Check sheet for the modelled part. Datum: model origin and axes. Units: mm. Face numbers are marked on the shaded views. A direction names the side the tool comes from. Coordinates: 2 decimals unless noted, no trailing zeros. Write each loop counter-clockwise with the first axis right and the second up, starting at its lowest first coordinate (ties: lowest second). Pieces come first, ordered by that corner, then holes. Notation, with made-up numbers: (74.5, 49) -> (109.5, 49) arc R13 ccw to (109.5, 56) -> close; hole circle Ø1 at (87.5, -4). An arc over 180 degrees is marked (long way). Put each result on its own line as item: value.
```python
from build123d import *

# Parameters (mm, degrees)
SKETCH033_W     = 136
SKETCH033_H     = 30
PAD012_DEPTH    = 10
SKETCH032_W     = 15
SKETCH032_H     = 30
PAD011_DEPTH    = 22
SKETCH030_W     = 30
SKETCH030_H     = 17
POCKET020_DEPTH = 10
SKETCH031_R     = 3
POCKET021_DEPTH = 10.001
SKETCH034_W     = 32.5
SKETCH034_H     = 30
POCKET022_DEPTH = 5
SKETCH040_R     = 5
POCKET028_DEPTH = 3
CHAMFER_SIZE2   = 25
CHAMFER_SIZE    = 10
CHAMFER010_SIZE = 1
SKETCH080_W     = 32.5
SKETCH080_H     = 9.75
PAD031_DEPTH    = 1
SKETCH084_R     = 3
POCKET051_DEPTH = 5


with BuildPart() as part:
    # Sketch033 → Pad012 (new body)
    with BuildSketch(Plane.XY):
        Rectangle(SKETCH033_W, SKETCH033_H)
    extrude(amount=PAD012_DEPTH)

    # Sketch032 (on Face5 of Pad012) → Pad011 (join)
    with BuildSketch(Plane(origin=(0, 0, 0), x_dir=(1, 0, 0), z_dir=(0, 0, -1))):
        with Locations((-60.5, 0)):
            Rectangle(SKETCH032_W, SKETCH032_H)
    extrude(amount=PAD011_DEPTH)

    # Sketch030 (on Face9 of Pad011) → Pocket020 (cut)
    with BuildSketch(Plane.YZ.offset(-53)):
        with Locations((0, -8.5)):
            Rectangle(SKETCH030_W, SKETCH030_H)
    extrude(amount=-POCKET020_DEPTH, mode=Mode.SUBTRACT)

    # Sketch031 (on Face5 of Pocket020) → Pocket021 (cut, through all)
    with BuildSketch(Plane(origin=(0, 0, 0), x_dir=(1, 0, 0), z_dir=(0, 0, -1))):
        with Locations((53, 0)):
            Circle(SKETCH031_R)
    extrude(amount=-POCKET021_DEPTH, mode=Mode.SUBTRACT)

    # Sketch034 → Pocket022 (cut)
    with BuildSketch(Plane.XY.offset(10)):
        with Locations((51.75, 0)):
            Rectangle(SKETCH034_W, SKETCH034_H)
    extrude(amount=-POCKET022_DEPTH, mode=Mode.SUBTRACT)

    # Sketch040 (on Face4 of Pocket022) → Pocket028 (cut)
    with BuildSketch(Plane(origin=(0, 0, 0), x_dir=(1, 0, 0), z_dir=(0, 0, -1))):
        with Locations((53, 0)):
            Circle(SKETCH040_R)
    extrude(amount=-POCKET028_DEPTH, mode=Mode.SUBTRACT)

    # Chamfer
    chamfer_edges = [part.edges().sort_by_distance(p)[0] for p in [
        (-53, 15, -19.5),
    ]]
    chamfer_side = part.faces().sort_by_distance((-63.15625, 15, -13.65625))[0]
    chamfer(chamfer_edges, length=CHAMFER_SIZE, length2=CHAMFER_SIZE2, reference=chamfer_side)

    # Chamfer010
    chamfer010_edges = [part.edges().sort_by_distance(p)[0] for p in [
        (-58, 2.5, -22),
        (-58, 2.5, -17),
        (-53, -12.5, -22),
        (-53, -12.5, -17),
        (-60.5, -15, -22),
        (-68, 0, -22),
        (-65.5, 15, -22),
        (-68, -15, -11),
        (-68, -15, 5),
        (-68, 0, 10),
        (-68, 15, 5),
        (-68, 15, -11),
    ]]
    chamfer(chamfer010_edges, length=CHAMFER010_SIZE)

    # Sketch080 (on Face21 of Chamfer010) → Pad031 (join)
    with BuildSketch(Plane.XY.offset(5)):
        with Locations((51.75, 0)):
            Rectangle(SKETCH080_W, SKETCH080_H)
    extrude(amount=PAD031_DEPTH)

    # Sketch084 (on Face33 of Pad031) → Pocket051 (cut)
    with BuildSketch(Plane.XY.offset(6)):
        with Locations((53, 0)):
            Circle(SKETCH084_R)
    extrude(amount=-POCKET051_DEPTH, mode=Mode.SUBTRACT)


solid = part.part
```
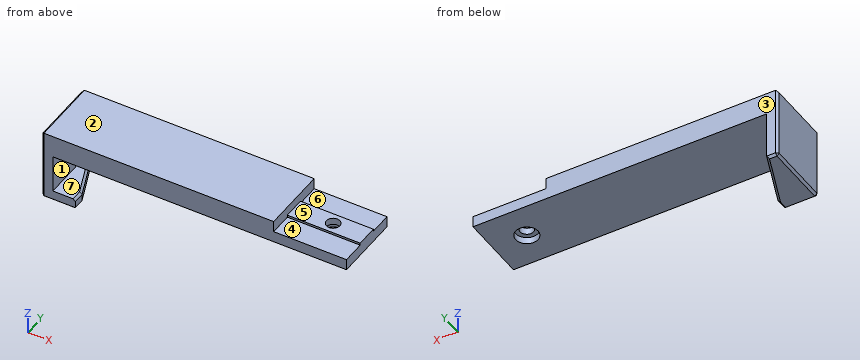
Q1. Depth check by flat-ended pin: P1, Ø5.5, axis at y = -5, z = -12, coming from the +X side; P2, Ø8, axis at x = 53, y = 2, coming from the -Z side; P3, Ø5, axis at x = 51.5, y = 9.5, coming from the +Z side. Enter the tip coordinate at first touch or a pass-through.
Recorded:
P1: stops at x = -63
P2: stops at z = 0
P3: stops at z = 5
Q2. Cross-section at A-A (x = 53). Record the cut outline in (y, z) (3 decimals).
Recorded:
outline: (-15, 0) -> (-5, 0) -> (-5, 3) -> (-3, 3) -> (-3, 6) -> (-4.875, 6) -> (-4.875, 5) -> (-15, 5) -> close; (3, 3) -> (5, 3) -> (5, 0) -> (15, 0) -> (15, 5) -> (4.875, 5) -> (4.875, 6) -> (3, 6) -> close
Q3. Material ranges on line 1 along Y through (x, z) = (53, 4); line 2 along Y through (x, z) = (53, 1); line 3 along X through (y, z) = (0, 4), recorded low to high.
Recorded:
line 1: y = -15 to -3, 3 to 15
line 2: y = -15 to -5, 5 to 15
line 3: x = -68 to 50, 56 to 68
Q4. Cross-section at D-D (z = -8). Record the cut outline in (x, y), plus the area to 3 significant figures.
Recorded:
outline: (-68, -14) -> (-67, -15) -> (-63, -15) -> (-63, 15) -> (-67, 15) -> (-68, 14) -> close
area: 149 mm2
Q5. Tool access check on the marked faces 4, 5, 6 and 7. Record the directions out of +Z, -Z, +X, -X, +Y, -Y that give a thin tool (end or side, any length) a straight path to the whole face; none if there is none.
Recorded:
face 4: +Z, +X, -Y
face 5: +Z, +X, +Y, -Y
face 6: +Z, +X, +Y
face 7: +X, +Y, -Y
Q6. Mould release check, pull along Z, two halves, no side actions. Record for the marked faces 1, 2 and 3: released by +Z, released by -Z, zero draft, split by the parting line, or undercut.
Recorded:
face 1: undercut
face 2: released by +Z
face 3: zero draft
Q7. Cross-section at C-C (y = 0). Record the cut outline in (x, z), plus the area to 3 significant figures.
Recorded:
outline: (-68, -21) -> (-67, -22) -> (-58.08, -22) -> (-57, -21) -> (-57, -18) -> (-58.08, -17) -> (-63, -17) -> (-63, 0) -> (48, 0) -> (48, 3) -> (50, 3) -> (50, 6) -> (35.5, 6) -> (35.5, 10) -> (-67, 10) -> (-68, 9) -> close; (56, 3) -> (58, 3) -> (58, 0) -> (68, 0) -> (68, 6) -> (56, 6) -> close
area: 1,320 mm2
Q8. Cross-section at B-B (y = -12). Record the cut outline in (x, z), plus the area to 3 significant figures.
Recorded:
outline: (-68, -21) -> (-67, -22) -> (-54, -22) -> (-53, -21) -> (-53, -18) -> (-54, -17) -> (-63, -17) -> (-63, 0) -> (68, 0) -> (68, 5) -> (35.5, 5) -> (35.5, 10) -> (-67, 10) -> (-68, 9) -> close
area: 1,360 mm2
